Geometry: final body of the model. Coordinates: model frame, mm. A direction names the side the tool comes from. Coordinates: 2 decimals unless noted, no trailing zeros. Loops run counter-clockwise (first coordinate to the right, second up) from the corner with the lowest first, then second, coordinate; pieces in that order, holes last. Notation, with made-up numbers: (-26.5, 61) - (13.5, 61) arc R19 ccw to (13.5, 91) - close; hole circle Ø2 at (69, 41). An arc over 180 degrees is marked (long way). Return JSON: item names as keys, results as strings.
from build123d import *

# Parameters (mm, degrees)
SKETCH1_W               = 27.54
SKETCH1_H               = 6
BOSS_EXTRUDE1_DEPTH     = 13
SKETCH2_R               = 1.65
CUT_EXTRUDE1_DEPTH      = 20.86486597
SKETCH4_W               = 27.54
SKETCH4_H               = 6
BOSS_EXTRUDE2_DEPTH     = 6
FILLET1_R               = 4
FILLET2_R               = 3
CUT_EXTRUDE2_DEPTH      = 20.86486597
CUT_EXTRUDE2_DEPTH_BACK = 20.86486597
SKETCH3_R               = 1.65
CUT_EXTRUDE3_DEPTH      = 4


with BuildPart() as part:
    # Sketch1 → Boss-Extrude1 (new body)
    with BuildSketch(Plane.XY):
        Rectangle(SKETCH1_W, SKETCH1_H)
    extrude(amount=BOSS_EXTRUDE1_DEPTH)

    # Sketch2 → Cut-Extrude1 (cut, through all)
    with BuildSketch(Plane(origin=(0, 3, 0), x_dir=(1, 0, 0), z_dir=(0, 1, 0))):
        with Locations(Location((-10.65, -6.5, 0), (0, 0, 270))):
            Circle(SKETCH2_R)
        with Locations(Location((10.65, -6.5, 0), (0, 0, 270))):
            Circle(SKETCH2_R)
    extrude(amount=-CUT_EXTRUDE1_DEPTH, mode=Mode.SUBTRACT)

    # Sketch4 → Boss-Extrude2 (add)
    with BuildSketch(Plane(origin=(0, 0, 0), x_dir=(-1, 0, 0), z_dir=(0, 0, -1))):
        Rectangle(SKETCH4_W, SKETCH4_H)
    extrude(amount=BOSS_EXTRUDE2_DEPTH)

    # Fillet1
    fillet1_edges = [part.edges().sort_by_distance(p)[0] for p in [
        (-13.77, 0, 13),
        (13.77, 0, 13),
    ]]
    fillet(fillet1_edges, radius=FILLET1_R)

    # Fillet2
    fillet2_edges = [part.edges().sort_by_distance(p)[0] for p in [
        (13.77, 0, -6),
        (-13.77, 0, -6),
    ]]
    fillet(fillet2_edges, radius=FILLET2_R)

    # Sketch3 → Cut-Extrude2 (cut, two sides: drawn at the far end of the back side and taken through both)
    with BuildSketch(Plane.XZ.offset(3).offset(-CUT_EXTRUDE2_DEPTH_BACK)):
        with Locations(Location((8.73, -3, 0), (0, 0, 270))):
            Circle(SKETCH3_R)
        with Locations(Location((-10.27, -3, 0), (0, 0, 270))):
            Circle(SKETCH3_R)
    extrude(amount=CUT_EXTRUDE2_DEPTH + CUT_EXTRUDE2_DEPTH_BACK, mode=Mode.SUBTRACT)

    # Sketch6 → Cut-Extrude3 (cut)
    with BuildSketch(Plane.XZ.offset(3)):
        Polygon((12.295448267, 9.35), (15.295448267, 9.35), (15.295448267, 3.65), (12.295448267, 3.65), (9.004551733, 3.65), (7.359103466, 6.5), (9.004551733, 9.35), align=None)
        Polygon((-12.295448267, 3.65), (-9.004551733, 3.65), (-7.359103466, 6.5), (-9.004551733, 9.35), (-12.295448267, 9.35), (-15.295448267, 9.35), (-15.295448267, 3.65), align=None)
    extrude(amount=-CUT_EXTRUDE3_DEPTH, mode=Mode.SUBTRACT)


solid = part.part
Item 1: First-contact query: pin 1 Ø2 at (y, z) = (-1, 9) entering from +X; pin 2 Ø5.5 at (x, z) = (10.65, 6.5) entering from -Y; pin 3 Ø2.5 at (x, z) = (-10.65, 6.5) entering from +Y. Flat tips, straight axial feed; report the tip coordinate or a pass-through.
Worked out:
{"pin 1": "x = 13.75", "pin 2": "y = 1", "pin 3": "through"}
Item 2: Reachability of faces 1 (the face through (-12, 1, 5)), 2 (the face through (8.17, -1.028, 7.905)), 3 (the face through (12.629, 0.042, 11.797)) from +Z, -Z, +X, -X, +Y, -Y: full face, straight path, thin tool, end or side. Return the list, or none.
Worked out:
{"face 1": "-X, -Y", "face 2": "+X, -Y", "face 3": "+Z, +X, +Y, -Y"}
Item 3: Ray query, probe 1 along X at (y, z) = (2.65, 6.5); probe 2 along X at (y, z) = (0.85, -3); probe 3 along Z at (x, y) = (8.73, 1.7). Return the intervals inside material, ascending. Write a range as from..to.
Worked out:
{"probe 1": "-13.77..-12.3, -9..9, 12.3..13.77", "probe 2": "-13.77..-11.92, -8.62..7.08, 10.38..13.77", "probe 3": "-6..-4.65, -1.35..13"}
Item 4: Section query D-D, the plane z = 10.75. Return loops of the section in (x, y), and give its area (3 significant figures).
Worked out:
{"outline": "(-13.37, -3) - (13.37, -3) - (13.37, 3) - (-13.37, 3) - close", "area": "160 mm^2"}
Item 5: Section query B-B, the plane x = -10.27. Return loops of the section in (y, z), and give its area (3 significant figures).
Worked out:
{"outline": "(-3, -6) - (3, -6) - (3, -4.65) - (-3, -4.65) - close; (-3, -1.35) - (3, -1.35) - (3, 4.89) - (1, 4.89) - (1, 3.65) - (-3, 3.65) - close; (-3, 9.35) - (1, 9.35) - (1, 8.11) - (3, 8.11) - (3, 12.97) - (-3, 12.97) - close", "area": "64.8 mm^2"}
Item 6: Section query A-A, the plane y = -2.6. Return loops of the section in (x, z).
Worked out:
{"outline": "(-13.77, -3) arc R3 ccw to (-10.77, -6) - (10.77, -6) arc R3 ccw to (13.77, -3) - (13.77, 3.65) - (9, 3.65) - (7.36, 6.5) - (9, 9.35) - (13.75, 9.35) arc R4 ccw to (9.77, 13) - (-9.77, 13) arc R4 ccw to (-13.75, 9.35) - (-9, 9.35) - (-7.36, 6.5) - (-9, 3.65) - (-13.77, 3.65) - close; hole circle Ø3.3 at (-10.27, -3); hole circle Ø3.3 at (8.73, -3)"}
Item 7: Section query C-C, the plane y = 1.6. Return loops of the section in (x, z), and give its area (3 significant figures).
Worked out:
{"outline": "(-13.77, -3) arc R3 ccw to (-10.77, -6) - (10.77, -6) arc R3 ccw to (13.77, -3) - (13.77, 9) arc R4 ccw to (9.77, 13) - (-9.77, 13) arc R4 ccw to (-13.77, 9) - close; hole circle Ø3.3 at (-10.65, 6.5); hole circle Ø3.3 at (-10.27, -3); hole circle Ø3.3 at (8.73, -3); hole circle Ø3.3 at (10.65, 6.5)", "area": "478 mm^2"}
